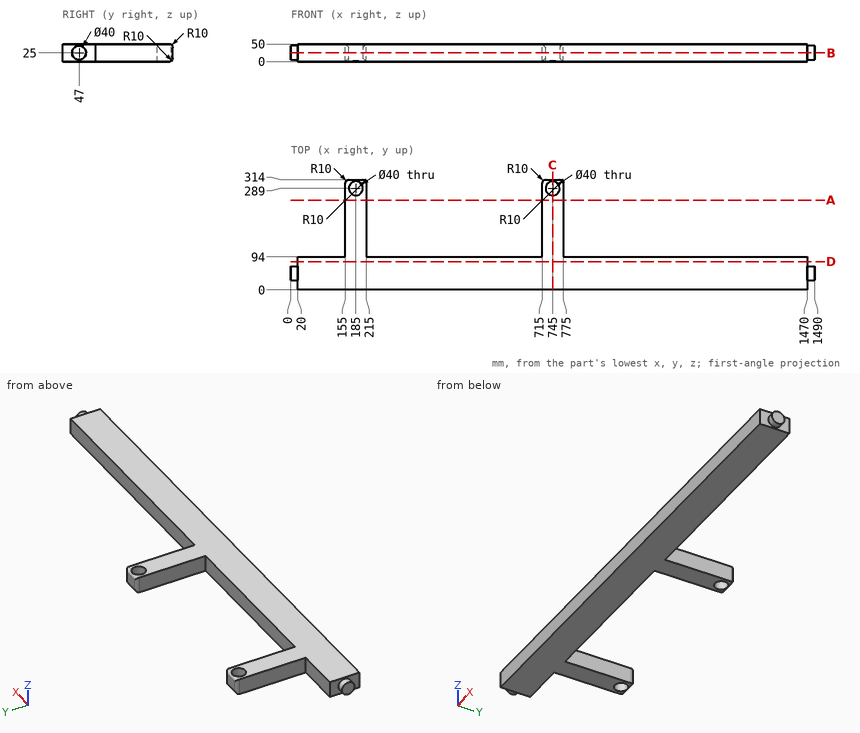
The figure shows three views and two pictorial views of one solid part (mm, origin at its lowest corner). Answer the questions. Round coordinates to 2 decimals unless told otherwise and drop trailing zeros. Order: outer loops, then holes, each group sorted by start corner. A loop starts at its lowest first (then second) coordinate and runs counter-clockwise, first axis right, second up. Notation, with made-up numbers: (87, 26) -> (92, 26) arc R29 cw to (92, 63) -> close; hole circle Ø7 at (82.5, 57). An arc over 180 degrees is marked (long way). Put each result on its own line as item: value.
Q1. Section C-C, the plane x = 745 is taken. Write down the section's boundary in (y, z), and give its area (3 significant figures).
Results list:
outline: (0, 0) -> (269, 0) -> (269, 50) -> (0, 50) -> close; (309, 1.34) arc R10 ccw to (314, 10) -> (314, 40) arc R10 ccw to (309, 48.66) -> close
area: 13,700 mm^2
Q2. Section B-B, the plane z = 25 is taken. Write down the section's boundary in (x, y), and give its area (3 significant figures).
Results list:
outline: (0, 27) -> (20, 27) -> (20, 0) -> (1470, 0) -> (1470, 27) -> (1490, 27) -> (1490, 67) -> (1470, 67) -> (1470, 94) -> (775, 94) -> (775, 304) arc R10 ccw to (765, 314) -> (725, 314) arc R10 ccw to (715, 304) -> (715, 94) -> (215, 94) -> (215, 304) arc R10 ccw to (205, 314) -> (165, 314) arc R10 ccw to (155, 304) -> (155, 94) -> (20, 94) -> (20, 67) -> (0, 67) -> close; hole circle Ø40 at (185, 289); hole circle Ø40 at (745, 289)
area: 162,000 mm^2
Q3. Consider line 1 along X through (y, z) = (289, 19.5); line 2 along X through (y, z) = (261.5, 36); line 3 along X through (y, z) = (275, 7). Determine where each line is inside the solid, lowest interval first.
Results list:
line 1: 155 to 165, 205 to 215, 715 to 725, 765 to 775
line 2: 155 to 215, 715 to 775
line 3: 155 to 170.72, 199.28 to 215, 715 to 730.72, 759.28 to 775
Q4. Section D-D, the plane y = 80.5 is taken. Write down the section's boundary in (x, z).
Results list:
outline: (20, 0) -> (1470, 0) -> (1470, 50) -> (20, 50) -> close
Q5. Each of these flat-tipped pins is pushed along its axis until it touches: P1, Ø15, axis at y = 204.5, z = 30, coming from the +X side; P2, Ø1, axis at y = 135, z = 15.5, coming from the -X side; P3, Ø12, axis at x = 702.5, z = 16, coming from the +Y side. Where does it stop, or does it pass through?
Results list:
P1: x = 775
P2: x = 155
P3: y = 94
Q6. Section A-A, the plane y = 255.5 is taken. Write down the section's boundary in (x, z), and give its area (3 significant figures).
Results list:
outline: (155, 0) -> (215, 0) -> (215, 50) -> (155, 50) -> close; (715, 0) -> (775, 0) -> (775, 50) -> (715, 50) -> close
area: 6,000 mm^2
